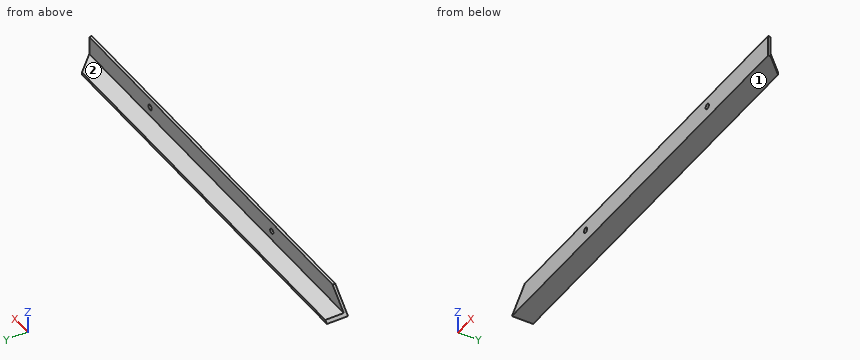
from build123d import *

# Parameters (mm, degrees)
SKETCH1_W           = 508
SKETCH1_H           = 25.4
BOSS_EXTRUDE1_DEPTH = 3.175
SKETCH2_W           = 508
SKETCH2_H           = 3.175
BOSS_EXTRUDE2_DEPTH = 22.225
CUT_EXTRUDE4_REACH  = 511.268
CUT_EXTRUDE5_DEPTH  = 22.225
SKETCH9_R           = 3.175
CUT_EXTRUDE6_DEPTH  = 3.175


with BuildPart() as part:
    # Sketch1 → Boss-Extrude1 (new body)
    with BuildSketch(Plane(origin=(0, 0, 0), x_dir=(1, 0, 0), z_dir=(0, 1, 0))):
        with Locations((-254, -12.7)):
            Rectangle(SKETCH1_W, SKETCH1_H)
    extrude(amount=BOSS_EXTRUDE1_DEPTH)

    # Sketch2 → Boss-Extrude2 (add)
    with BuildSketch(Plane(origin=(0, 3.175, 0), x_dir=(1, 0, 0), z_dir=(0, 1, 0))):
        with Locations((-254, -1.5875)):
            Rectangle(SKETCH2_W, SKETCH2_H)
    extrude(amount=BOSS_EXTRUDE2_DEPTH)

    # Cut-Extrude4: up to this face of the body (flat: up to its plane)
    cut_extrude4_end = Plane(part.part.faces().sort_by_distance((-254, 0, 12.7))[0])
    # Sketch7 → Cut-Extrude4 (cut, up to the picked face)
    with BuildSketch(Plane(origin=(0, 25.4, 0), x_dir=(1, 0, 0), z_dir=(0, 1, 0)), mode=Mode.PRIVATE) as cut_extrude4_sk1:
        Polygon((-508, 0), (-465.114238784, -42.885761216), (-525.028652123, -42.885761216), align=None)
    cut_extrude4_tool1 = split(extrude(cut_extrude4_sk1.sketch, amount=-CUT_EXTRUDE4_REACH, mode=Mode.PRIVATE), bisect_by=cut_extrude4_end, keep=Keep.BOTH, mode=Mode.PRIVATE)
    add(cut_extrude4_tool1.solids().sort_by(Axis((-499.380964, 25.4, 28.590507), (0, -1, 0)))[0], mode=Mode.SUBTRACT)

    # Sketch8 → Cut-Extrude5 (cut)
    with BuildSketch(Plane.XY.offset(3.175)):
        Polygon((0, 3.175), (-40.651364309, 43.826364309), (40.603016419, 27.12928401), align=None)
    extrude(amount=-CUT_EXTRUDE5_DEPTH, mode=Mode.SUBTRACT)

    # Sketch9 → Cut-Extrude6 (cut)
    with BuildSketch(Plane(origin=(0, 3.175, 0), x_dir=(1, 0, 0), z_dir=(0, 1, 0))):
        with Locations(Location((-361.95, -14.2875, 0), (0, 0, 270))):
            Circle(SKETCH9_R)
        with Locations(Location((-120.65, -14.2875, 0), (0, 0, 90))):
            Circle(SKETCH9_R)
    extrude(amount=-CUT_EXTRUDE6_DEPTH, mode=Mode.SUBTRACT)


solid = part.part
Source: CAD feature listing. Evaluate the final solid. Frame: model axes, mm. Face numbers are marked on the shaded views. A direction names the side the tool comes from. Round coordinates to 2 decimals unless told otherwise and drop trailing zeros. Loops run counter-clockwise (first coordinate to the right, second up) from the corner with the lowest first, then second, coordinate; pieces in that order, holes last. Notation, with made-up numbers: (65, 71) - (69, 71) arc R28 ccw to (69, 94) - close; hole circle Ø9 at (21.25, -9.75). An arc over 180 degrees is marked (long way). Write item = value, one per line. Start each with the question number.
Item 1: Material intervals for line 1 (Z direction, x = -361.95, y = 2); line 2 (Z direction, x = -411.5, y = 5.5) (3 decimals), sorted ascending.
Item 2: First-contact query: pin 1 Ø1.5 at (x, z) = (-78.5, 12.5) entering from +Y (3 decimals); pin 2 Ø8 at (y, z) = (20, 8) entering from -X; pin 3 Ø11 at (x, y) = (-146, 17.5) entering from +Z (3 decimals). Flat tips, straight axial feed; report the tip coordinate or a pass-through.
Item 3: Section query A-A on x = -476. Output: boundary loops of the cut face in (y, z) (3 decimals), plus the area to 3 significant figures.
Item 4: Reachability of the marked faces 1 and 2 from +Z, -Z, +X, -X, +Y, -Y: full face, straight path, thin tool, end or side. Return the list, or none.
Item 5: Section query B-B on y = 14. Output: boundary loops of the cut face in (x, z) (3 decimals), plus the area to 3 significant figures.
Results list:
q1.line_1 = 0 to 11.11, 17.46 to 25.4
q1.line_2 = 0 to 3.175
q2.pin_1 = 3.175
q2.pin_2 = through
q2.pin_3 = 3.175
q3.outline = (0, 0) - (25.4, 0) - (25.4, 3.175) - (3.175, 3.175) - (3.175, 25.4) - (0, 25.4) - close
q3.area = 151 mm²
q4.face_1 = -Z, +X, -X, +Y, -Y
q4.face_2 = +Z, +X, -X, +Y
q5.outline = (-508, 0) - (-10.825, 0) - (-10.825, 3.175) - (-504.825, 3.175) - close
q5.area = 1,570 mm²
